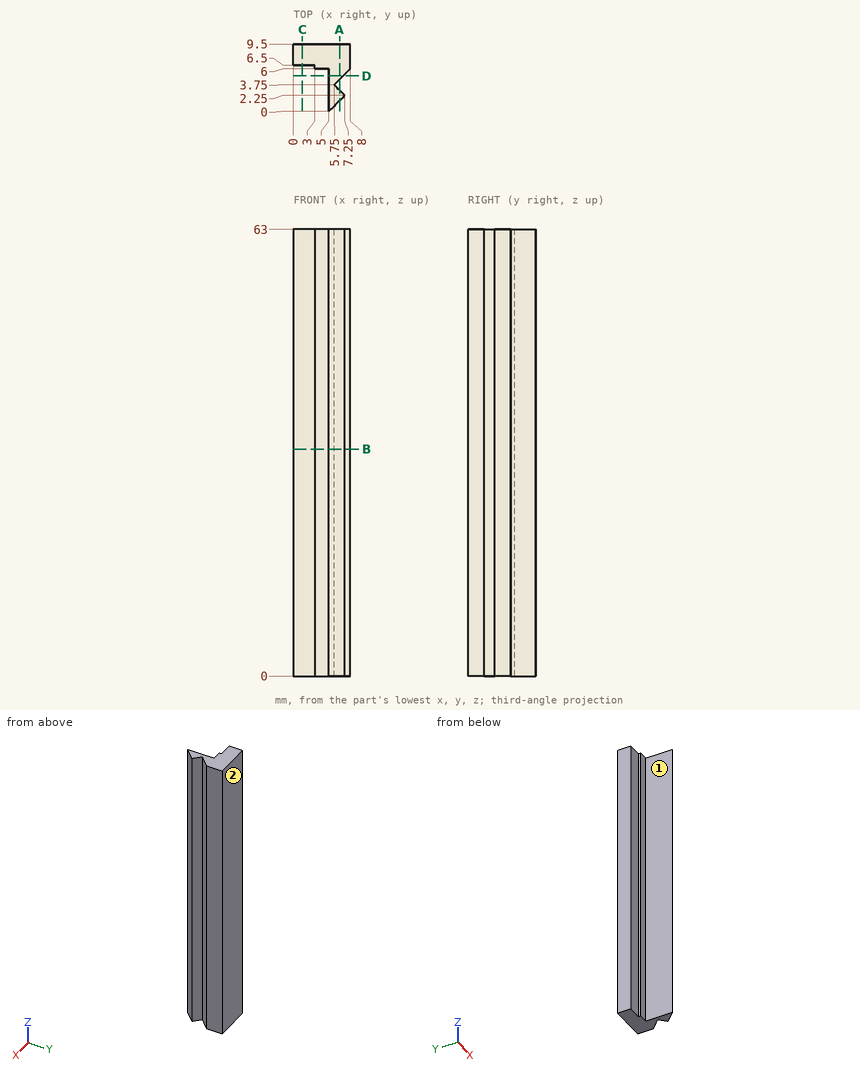
Geometry check sheet. Reference: drawing and pictorial views, mm from the part's lowest x, y, z. A direction names the side the tool comes from. Coordinates: 2 decimals unless noted, no trailing zeros. Order: outer loops, then holes, each group sorted by start corner. A loop starts at its lowest first (then second) coordinate and runs counter-clockwise, first axis right, second up.
1. Scan lines: line 1 (X direction, y = 3.5, z = 13.5); line 2 (Y direction, x = 1.25, z = 49); line 3 (Y direction, x = 4, z = 20). Record each from-to range of solid material in increasing order.
Results found:
line 1: x = 5 to 6
line 2: y = 6.5 to 9.5
line 3: y = 6 to 9.5
2. Sectioned sample at B-B, the plane z = 32. Record the cut outline in (x, y).
Results found:
outline: (0, 6.5) - (3, 6.5) - (3, 6) - (5, 6) - (5, 0) - (7.25, 2.25) - (5.75, 3.75) - (8, 6) - (8, 9.5) - (0, 9.5) - close
3. Go/stop test with flat-tipped pins: pin 1 Ø0.9 at (x, z) = (1.5, 35) entering from -Y; pin 2 Ø1.6 at (x, z) = (4.5, 16.5) entering from -Y; pin 3 Ø2 at (y, z) = (3.5, 16.5) entering from -X. Record where each tip stops, or that it passes through.
Results found:
pin 1: stops at y = 6.5
pin 2: stops at y = 0
pin 3: stops at x = 5
4. Sectioned sample at C-C, the plane x = 1.25. Record the cut outline in (y, z), and give its area (3 significant figures).
Results found:
outline: (6.5, 0) - (9.5, 0) - (9.5, 63) - (6.5, 63) - close
area: 189 mm2
5. Sectioned sample at A-A, the plane x = 6.5. Record the cut outline in (y, z).
Results found:
outline: (1.5, 0) - (3, 0) - (3, 63) - (1.5, 63) - close; (4.5, 0) - (9.5, 0) - (9.5, 63) - (4.5, 63) - close
6. Sectioned sample at D-D, the plane y = 5. Record the cut outline in (x, z).
Results found:
outline: (5, 0) - (7, 0) - (7, 63) - (5, 63) - close
7. Set-up check for the marked faces 1 and 2: record each of +Z, -Z, +X, -X, +Y, -Y from which the full face is reachable in a straight line by a thin tool's end or side.
Results found:
face 1: +Z, -Z, -X, -Y
face 2: +Z, -Z, +X, -X, +Y
